Geometry: see drawing. Coordinates: mm, zero at the bounding-box minimum. Coordinates: 2 decimals unless noted, no trailing zeros. Order: outer loops, then holes, each group sorted by start corner. A loop starts at its lowest first (then second) coordinate and runs counter-clockwise, first axis right, second up.
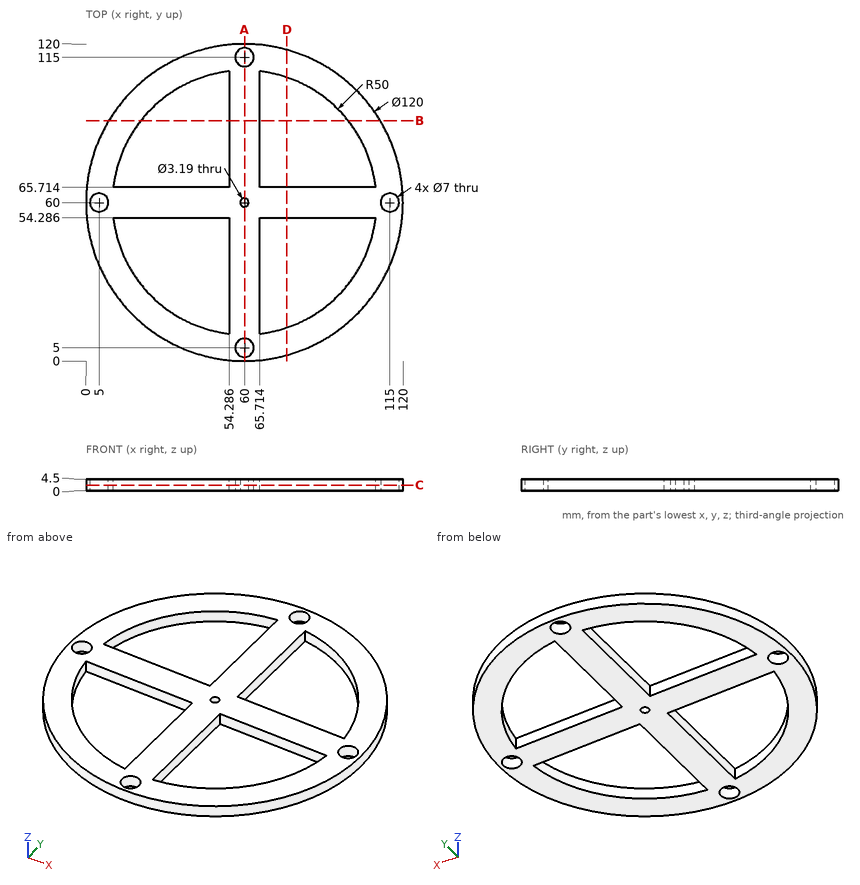
Q1. Section query A-A on x = 60. Output: boundary loops of the cut face in (y, z) (1 decimal).
Solutions:
outline: (0, 0) - (1.5, 0) - (1.5, 4.5) - (0, 4.5) - close; (8.5, 0) - (58.4, 0) - (58.4, 4.5) - (8.5, 4.5) - close; (61.6, 0) - (111.5, 0) - (111.5, 4.5) - (61.6, 4.5) - close; (118.5, 0) - (120, 0) - (120, 4.5) - (118.5, 4.5) - close
Q2. Section query B-B on y = 91. Output: boundary loops of the cut face in (x, z), plus the area to 3 significant figures.
Solutions:
outline: (8.63, 0) - (20.77, 0) - (20.77, 4.5) - (8.63, 4.5) - close; (54.29, 0) - (65.71, 0) - (65.71, 4.5) - (54.29, 4.5) - close; (99.23, 0) - (111.37, 0) - (111.37, 4.5) - (99.23, 4.5) - close
area: 161 mm2
Q3. Section query C-C on z = 2.2. Give the number of separate pieces and of enclosed holes in the cut face, plus the area to 3 significant figures.
Solutions:
separate pieces: 1
enclosed holes: 9
area: 5,440 mm2
Q4. Material intervals for line 1 along Y through (x, z) = (60, 2.2) (1 decimal); line 2 along Y through (x, z) = (48, 2.85) (1 decimal), sorted ascending.
Solutions:
line 1: y = 0 to 1.5, 8.5 to 58.4, 61.6 to 111.5, 118.5 to 120
line 2: y = 1.2 to 11.5, 54.3 to 65.7, 108.5 to 118.8
Q5. Section query D-D on x = 76. Output: boundary loops of the cut face in (y, z).
Solutions:
outline: (2.17, 0) - (12.63, 0) - (12.63, 4.5) - (2.17, 4.5) - close; (54.29, 0) - (65.71, 0) - (65.71, 4.5) - (54.29, 4.5) - close; (107.37, 0) - (117.83, 0) - (117.83, 4.5) - (107.37, 4.5) - close
Q6. Pin query (flat end, axial travel): P1, Ø6.5, axis at x = 115, y = 60, coming from the +Z side; P2, Ø2, axis at y = 78.5, z = 1.5, coming from the +X side; P3, Ø1.5, axis at y = 35.5, z = 4, coming from the -X side; P4, Ø2, axis at x = 39, z = 2, coming from the +Y side. Return the tip coordinate at first contact, or that it passes through.
Solutions:
P1: passes through
P2: stops at x = 117.39
P3: stops at x = 4.9
P4: stops at y = 116.57
